Geometry check sheet. Reference: the model listing, model coordinates, mm. Face numbers are marked on the shaded views. A direction names the side the tool comes from. Coordinates: 2 decimals unless noted, no trailing zeros. Order: outer loops, then holes, each group sorted by start corner. A loop starts at its lowest first (then second) coordinate and runs counter-clockwise, first axis right, second up. Notation, with made-up numbers: M 7.5,-2 L 36.5,-2 A21 ccw 36.5,7 Z; hole C 70.25,58.25 d9. An arc over 180 degrees is marked long. One line per item, written item: value. Start each with the question number.
1) Thickness scan on L1, parallel to X at y = 0, z = 3.5; L2, parallel to Z at x = -2.5, y = 9.5; L3, parallel to X at y = 0, z = 1.1. Record the ranges inside material, lowest first. Write a range as from..to.
2) Access from +Z, -Z, +X, -X, +Y, -Y to the whole of each face (thin tool, end or side, straight path). Record for the marked faces 1, 2 and 3.
3) Go/stop test with flat-tipped pins: P1, Ø3.5, axis at x = -2.5, y = 14.79, coming from the +Z side; P2, Ø2.5, axis at x = 2.5, y = 8.029, coming from the +Z side; P3, Ø3, axis at y = 4.5, z = 3, coming from the -X side. Record where each tip stops, or that it passes through.
4) Sectioned sample at D-D, the plane z = 1.2. Enter the section's corners in (x, y), then the cut area to 3 significant figures.
5) Sectioned sample at B-B, the plane x = 2.5. Enter the section's corners in (y, z).
6) Sectioned sample at C-C, the plane z = 3.6. Enter the section's corners in (x, y).
7) Sectioned sample at A-A, the plane y = 0.25. Enter the section's corners in (x, z).
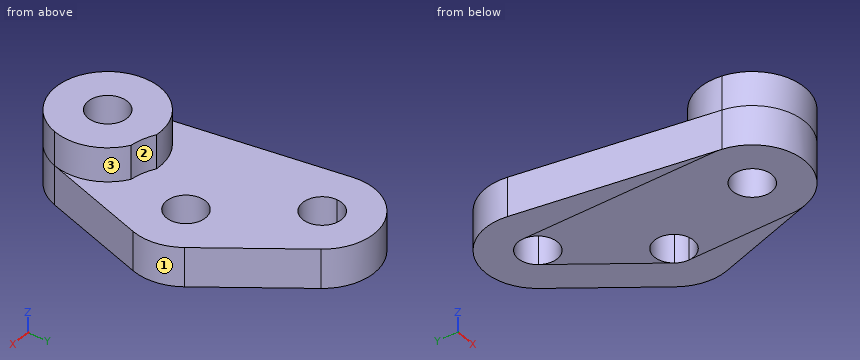
Autodesk Inventor part; units mm, degrees
ref_plane "YZ Plane" through (0, 0, 0) normal (1, 0, 0) x (0, 1, 0)
ref_plane "XZ Plane" through (0, 0, 0) normal (0, 1, 0) x (-1, 0, 0)
ref_plane "XY Plane" through (0, 0, 0) normal (0, 0, 1) x (1, 0, 0)
sketch "Skizze1" plane through (0, 0, 0) normal (0, 0, 1) x (1, 0, 0)
  circle A0 centre (0, 0) radius 4
  circle A1 centre (-2.5, 14.7902) radius 1.5
  circle A2 centre (2.5, 8.029) radius 1.5
  line L0 (-4, 0) -> (-4, 14.7902)
  line L1 (-1.294, 15.6821) -> (3.706, 8.9208)
  line L2 (4, 8.029) -> (4, 0)
  line L3 (0, 0) -> (-2.5, 14.7902) construction
  line L4 (2.5, 8.029) -> (-1.25, 7.3951) construction
  dimension "d0" = 8
  dimension "d1" = 3
  dimension "d3" = 15
extrude "Extrusion1" add sketch "Skizze1" along normal blind 3
sketch "Skizze2" plane through (0, 0, 3) normal (0, 0, 1) x (1, 0, 0)
  arc A0 (4, 8.029) -> (3.706, 8.9208) centre (2.5, 8.029) ccw
  arc A1 (-1.294, 15.6821) -> (-4, 14.7902) centre (-2.5, 14.7902) ccw
  arc A2 (-4, 0) -> (4, 0) centre (0, 0) ccw
hole "Bohrung1" at (2.5, 8.029, 3) at (-2.5, 14.7902, 3) at (0, 0, 3) direction (0, 0, -1) diameter 3 end through all
sketch "Skizze3" plane through (0, 0, 3) normal (0, 0, 1) x (1, 0, 0)
  circle A0 centre (-2.5, 14.7902) radius 1.5
  circle A1 centre (2.5, 8.029) radius 1.5
  arc A2 (4, 8.029) -> (3.706, 8.9208) centre (2.5, 8.029) ccw
  line L0 (3.706, 8.9208) -> (-1.294, 15.6821)
  arc A3 (-1.294, 15.6821) -> (-4, 14.7902) centre (-2.5, 14.7902) ccw
  line L1 (-4, 14.7902) -> (-4, 0)
  arc A4 (-4, 0) -> (4, 0) centre (0, 0) ccw
  line L2 (4, 0) -> (4, 8.029)
  arc A5 (0.7161, 17.1686) -> (-6.4441, 14.1235) centre (-2.5, 14.7902) ccw
  arc A6 (6.3191, 6.8398) -> (5.7161, 10.4073) centre (2.5, 8.029) ccw
  arc A7 (-3.9441, -0.6667) -> (3.8191, -1.1892) centre (0, 0) ccw
  line L3 (3.8191, -1.1892) -> (6.3191, 6.8398)
  line L4 (-3.9441, -0.6667) -> (-6.4441, 14.1235)
  line L5 (0.7161, 17.1686) -> (5.7161, 10.4073)
  circle A8 centre (0, 0) radius 1.5
  dimension "d13" = 2.5
  dimension "d14" = 2.5
  dimension "d24" = 2.5
extrude "Extrusion2" add sketch "Skizze3" against normal up to surface (3 mm away) contours A0 L1 A4 L4 A5 L5 A6 L3 L2 A1 L0
sketch "Skizze4" plane through (0, 0, 3) normal (0, 0, 1) x (1, 0, 0)
  arc A0 (6.3191, 6.8398) -> (5.7161, 10.4073) centre (2.5, 8.029) ccw
  arc A1 (0.7161, 17.1686) -> (-6.4441, 14.1235) centre (-2.5, 14.7902) ccw
  arc A2 (0.2281, 11.8649) -> (-0.5021, 11.3249) centre (2.5, 8.029) ccw
  arc A3 (0.2281, 11.8649) -> (0.7161, 17.1686) centre (-2.5, 14.7902) ccw
  arc A4 (-6.4441, 14.1235) -> (-0.5021, 11.3249) centre (-2.5, 14.7902) ccw
  circle A5 centre (2.5, 8.029) radius 1.5
  arc A6 (-3.9441, -0.6667) -> (3.8191, -1.1892) centre (0, 0) ccw
  arc A7 (0.2261, 3.9936) -> (2.081, 3.416) centre (0, 0) ccw
  arc A8 (0.2261, 3.9936) -> (2.081, 3.416) centre (2.5, 8.029) ccw
  circle A9 centre (0, 0) radius 1.5
extrude "Extrusion3" add sketch "Skizze4" along normal blind 2.6 contours A7 A8 A6
equation "\"d0\" = 2 * bearingWall"
equation "\"d1\" = bearingHole"
equation "\"d4\" = Join_width"
equation "\"d6\" = bearingHole"
equation "\"d13\" = d24"
equation "\"d14\" = d13"
equation "\"FingerLaenge_B\" = 25"
equation "\"Hebel_B\" = 25"
equation "\"Finger_width\" = 22"
equation "\"Finger_diameter\" = 8"
equation "\"FingerWall\" = 3"
equation "\"Hebel_basis_2\" = 15"
equation "\"Join_width\" = 3"
equation "\"bearingHole\" = 3"
equation "\"bearingWall\" = 4"
equation "\"support_D\" = 0.25"
properties part number "3_hebenMount_2_dual"
Final values:
1. L1: x = -4..-1.5, 1.5..4
1. L2: z = 0..3
1. L3: x = -4.06..-1.5, 1.5..4.19
2. face 1: +Z, -Z, +X
2. face 2: +Z, +X, +Y
2. face 3: +Z, +X
3. P1: stops at z = 3
3. P2: passes through
3. P3: stops at x = -5.07
4. outline: M -6.44,14.12 L -3.94,-0.67 A4 ccw 3.82,-1.19 L 6.32,6.84 A4 ccw 5.72,10.41 L 0.72,17.17 A4 ccw Z; hole C -2.5,14.79 d3; hole C 0,0 d3; hole C 2.5,8.03 d3
4. area: 185 mm^2
5. outline: M -3.12,0 L 6.53,0 L 6.53,3 L 3.12,3 L 3.12,5.6 L -3.12,5.6 Z; M 9.53,0 L 14.76,0 L 14.76,3 L 9.53,3 Z
6. outline: M -3.94,-0.67 A4 ccw 3.82,-1.19 A4 ccw 2.08,3.42 A4.63 cw 0.23,3.99 A4 ccw Z; hole C 0,0 d3
7. outline: M -4.1,0 L -1.48,0 L -1.48,5.6 L -3.99,5.6 L -3.99,3 L -4.1,3 Z; M 1.48,0 L 4.27,0 L 4.27,3 L 3.99,3 L 3.99,5.6 L 1.48,5.6 Z
